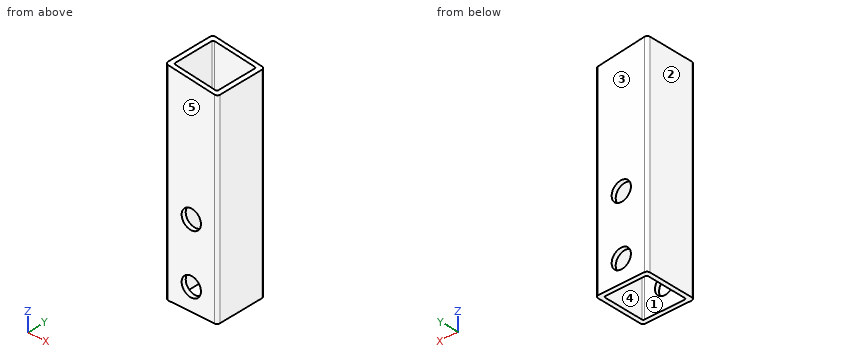
```python
from build123d import *

# Parameters (mm, degrees)
DODANIE_WYCI_GNI_CIE1_DEPTH = 140
SZKIC2_R                    = 6.5
WYTNIJ_WYCI_GNI_CIE1_DEPTH  = 140


with BuildPart() as part:
    # Szkic1 → Dodanie-wyciągnięcie1 (new body)
    with BuildSketch(Plane.XY):
        with BuildLine():
            Line((-15.5, 0), (15.5, 0))
            ThreePointArc((15.5, 0), (16.914213562, 0.585786438), (17.5, 2))
            Line((17.5, 2), (17.5, 33))
            ThreePointArc((17.5, 33), (16.914213562, 34.414213562), (15.5, 35))
            Line((15.5, 35), (-15.5, 35))
            ThreePointArc((-15.5, 35), (-16.914213562, 34.414213562), (-17.5, 33))
            Line((-17.5, 33), (-17.5, 2))
            ThreePointArc((-17.5, 2), (-16.914213562, 0.585786438), (-15.5, 0))
        make_face()
        with BuildLine():
            Line((-13.5, 3), (13.5, 3))
            ThreePointArc((13.5, 3), (14.207106781, 3.292893219), (14.5, 4))
            Line((14.5, 4), (14.5, 31))
            ThreePointArc((14.5, 31), (14.207106781, 31.707106781), (13.5, 32))
            Line((13.5, 32), (-13.5, 32))
            ThreePointArc((-13.5, 32), (-14.207106781, 31.707106781), (-14.5, 31))
            Line((-14.5, 31), (-14.5, 4))
            ThreePointArc((-14.5, 4), (-14.207106781, 3.292893219), (-13.5, 3))
        make_face(mode=Mode.SUBTRACT)
    extrude(amount=DODANIE_WYCI_GNI_CIE1_DEPTH)

    # Szkic2 → Wytnij-wyciągnięcie1 (cut)
    with BuildSketch(Plane(origin=(0, 35, 0), x_dir=(1, 0, 0), z_dir=(0, 1, 0))):
        with Locations(Location((0, -15, 0), (0, 0, 180))):
            Circle(SZKIC2_R)
        with Locations(Location((0, -55, 0), (0, 0, 180))):
            Circle(SZKIC2_R)
        Polygon((-17.5, -140), (23.891746827, -134.917732541), (23.891746827, -140), align=None)
    extrude(amount=-WYTNIJ_WYCI_GNI_CIE1_DEPTH, mode=Mode.SUBTRACT)


solid = part.part
```
Geometry check sheet. Reference: the model listing, model coordinates, mm. Face numbers are marked on the shaded views. A direction names the side the tool comes from. Round coordinates to 2 decimals unless told otherwise and drop trailing zeros. Loops run counter-clockwise (first coordinate to the right, second up) from the corner with the lowest first, then second, coordinate; pieces in that order, holes last. Notation, with made-up numbers: (28.5, 43.5) - (74.5, 43.5) arc R27 cw to (74.5, 67.5) - close; hole circle Ø9 at (52, 47.5). An arc over 180 degrees is marked (long way). Use a Markdown table: item, result.
Q1. Material ranges on line 1 (Y direction, x = -11, z = 127.5); line 2 (X direction, y = 9.5, z = 60.5); line 3 (Z direction, x = 0, y = 34.05), recorded low to high.
Solutions:
| item | result |
|---|---|
| line 1 | y = 0 to 3, 32 to 35 |
| line 2 | x = -17.5 to -14.5, 14.5 to 17.5 |
| line 3 | z = 0 to 8.5, 21.5 to 48.5, 61.5 to 137.85 |
Q2. Access from +Z, -Z, +X, -X, +Y, -Y to the whole of each face (thin tool, end or side, straight path). Record for the marked faces 1 and 2.
Solutions:
| item | result |
|---|---|
| face 1 | +Z, -Z |
| face 2 | +Z, -Z, -X, +Y, -Y |
Q3. Cross-section at A-A on y = 7.5. Record the cut outline in (x, z).
Solutions:
| item | result |
|---|---|
| outline | (-17.5, 0) - (-14.5, 0) - (-14.5, 139.63) - (-17.5, 140) - close; (14.5, 0) - (17.5, 0) - (17.5, 135.7) - (14.5, 136.07) - close |
Q4. Draft check along Y on the marked faces 3, 4 and 5. Enter one of: released by +Y, released by -Y, zero draft, split by the parting line, or undercut.
Solutions:
| item | result |
|---|---|
| face 3 | released by +Y |
| face 4 | undercut |
| face 5 | released by -Y |
Q5. Cross-section at D-D on z = 88. Record the cut outline in (x, y), plus the area to 3 significant figures.
Solutions:
| item | result |
|---|---|
| outline | (-17.5, 2) arc R2 ccw to (-15.5, 0) - (15.5, 0) arc R2 ccw to (17.5, 2) - (17.5, 33) arc R2 ccw to (15.5, 35) - (-15.5, 35) arc R2 ccw to (-17.5, 33) - close; hole (-14.5, 4) arc R1 ccw to (-13.5, 3) - (13.5, 3) arc R1 ccw to (14.5, 4) - (14.5, 31) arc R1 ccw to (13.5, 32) - (-13.5, 32) arc R1 ccw to (-14.5, 31) - close |
| area | 381 mm2 |
Q6. Go/stop test with flat-tipped pins: P1, Ø4, axis at x = -12, y = 25, coming from the -Z side; P2, Ø17, axis at x = 0, z = 15, coming from the +Y side. Record where each tip stops, or that it passes through.
Solutions:
| item | result |
|---|---|
| P1 | passes through |
| P2 | stops at y = 35 |
Q7. Cross-section at C-C on x = 3. Record the cut outline in (y, z), plus the area to 3 significant figures.
Solutions:
| item | result |
|---|---|
| outline | (0, 0) - (3, 0) - (3, 9.23) - (0, 9.23) - close; (0, 20.77) - (3, 20.77) - (3, 49.23) - (0, 49.23) - close; (0, 60.77) - (3, 60.77) - (3, 137.48) - (0, 137.48) - close; (32, 0) - (35, 0) - (35, 9.23) - (32, 9.23) - close; (32, 20.77) - (35, 20.77) - (35, 49.23) - (32, 49.23) - close; (32, 60.77) - (35, 60.77) - (35, 137.48) - (32, 137.48) - close |
| area | 687 mm2 |
Q8. Cross-section at B-B on z = 55. Record the cut outline in (x, y), plus the area to 3 significant figures.
Solutions:
| item | result |
|---|---|
| outline | (-17.5, 2) arc R2 ccw to (-15.5, 0) - (-6.5, 0) - (-6.5, 3) - (-13.5, 3) arc R1 cw to (-14.5, 4) - (-14.5, 31) arc R1 cw to (-13.5, 32) - (-6.5, 32) - (-6.5, 35) - (-15.5, 35) arc R2 ccw to (-17.5, 33) - close; (6.5, 0) - (15.5, 0) arc R2 ccw to (17.5, 2) - (17.5, 33) arc R2 ccw to (15.5, 35) - (6.5, 35) - (6.5, 32) - (13.5, 32) arc R1 cw to (14.5, 31) - (14.5, 4) arc R1 cw to (13.5, 3) - (6.5, 3) - close |
| area | 303 mm2 |
